Design review of the part built by this model. Coordinates are the model's own, in mm. Face numbers are marked on the shaded views. A direction names the side the tool comes from. Round coordinates to 2 decimals unless told otherwise and drop trailing zeros. Loops run counter-clockwise (first coordinate to the right, second up) from the corner with the lowest first, then second, coordinate; pieces in that order, holes last. Notation, with made-up numbers: (79, -8) - (136, -8) arc R12 cw to (136, 3) - close; hole circle Ø5 at (22, 81). An arc over 180 degrees is marked (long way). Use one line per item in the form item = value. Start each with the question number.
(1) We need section D-D, the plane z = -0.75. Write out the cut boundary in (x, y) (3 decimals).
(2) The part is to be moulded in two halves that separate along X. For the marked faces 3, 4, 5 and 6, say which applies: released by +X, released by -X, zero draft, split by the parting line, or undercut.
(3) We need section C-C, the plane z = 1. Write out the cut boundary in (x, y).
(4) We need section B-B, the plane x = 0. Write out the cut boundary in (y, z) (3 decimals).
(5) We need section A-A, the plane y = 0. Write out the cut boundary in (x, z) (3 decimals).
(6) For pin 1 (1.5 mm diameter, centred on x = -4.5, y = 2, fed in from +Z), flat-tipped, find the tip position at first contact; note if it passes through.
(7) Machinability: for the marked faces 1 and 2, which of the approach directions +Z, -Z, +X, -X, +Y, -Y give a long, thin tool a straight path to every point of the face, cutting with its end or side? Answer none if there is none.
(8) Wall thickness on probe 1 along Y at (x, z) = (0, -1.05) (3 decimals); probe 2 along Z at (x, y) = (-0.5, -2.75); probe 3 along X at (y, z) = (4.25, 1.75): over which ranges is each line inside the solid? List them lowest first. Write a range as [from, to].
Autodesk Inventor part; units mm, degrees
ref_plane "YZ Plane" through (0, 0, 0) normal (1, 0, 0) x (0, 1, 0)
ref_plane "XZ Plane" through (0, 0, 0) normal (0, 1, 0) x (-1, 0, 0)
ref_plane "XY Plane" through (0, 0, 0) normal (0, 0, 1) x (1, 0, 0)
sketch "Sketch1" plane through (0, 0, 0) normal (0, 0, 1) x (1, 0, 0)
  circle A0 centre (0, 0) radius 2.075
  line L0 (-12.5, 5) -> (12.5, 5)
  line L1 (12.5, 5) -> (12.5, -5)
  line L2 (12.5, -5) -> (-12.5, -5)
  line L3 (-12.5, -5) -> (-12.5, 5)
  line L4 (-12.5, 5) -> (12.5, -5) construction
  line L5 (12.5, 5) -> (-12.5, -5) construction
  dimension "d0" = 4.15
  dimension "d1" = 25
  dimension "d2" = 10
extrude "Extrusion1" add sketch "Sketch1" against normal blind 3.5
sketch "Sketch3" plane through (0, 0, 0) normal (0, 0, 1) x (1, 0, 0)
  line L0 (-22.7487, 17.0919) -> (-7.9081, 2.2513)
  arc A0 (-7.3223, 0.837) -> (-7.9081, 2.2513) centre (-9.3223, 0.837) ccw
  line L1 (-7.3223, 0.837) -> (-7.3223, -0.837)
  arc A1 (-7.9081, -2.2513) -> (-7.3223, -0.837) centre (-9.3223, -0.837) ccw
  line L2 (-7.9081, -2.2513) -> (-22.7487, -17.0919)
  line L3 (22.7487, -17.0919) -> (7.9081, -2.2513)
  arc A2 (7.3223, -0.837) -> (7.9081, -2.2513) centre (9.3223, -0.837) ccw
  line L4 (7.3223, -0.837) -> (7.3223, 0.837)
  arc A3 (7.9081, 2.2513) -> (7.3223, 0.837) centre (9.3223, 0.837) ccw
  line L5 (7.9081, 2.2513) -> (22.7487, 17.0919)
  circle A4 centre (0, 0) radius 1.65
  line L6 (-22.7487, 17.0919) -> (-22.7487, -17.0919)
  line L7 (22.7487, 17.0919) -> (22.7487, -17.0919)
  line L8 (-8.0495, 2.1098) -> (-22.5487, 16.609)
  line L9 (-22.5487, 16.609) -> (-22.5487, -16.609)
  line L10 (-22.5487, -16.609) -> (-8.0495, -2.1098)
  arc A5 (-7.5223, 0.837) -> (-8.0495, 2.1098) centre (-9.3223, 0.837) ccw
  line L11 (-7.5223, 0.837) -> (-7.5223, -0.837)
  arc A6 (-8.0495, -2.1098) -> (-7.5223, -0.837) centre (-9.3223, -0.837) ccw
  line L12 (7.5223, -0.837) -> (7.5223, 0.837)
  arc A7 (8.0495, 2.1098) -> (7.5223, 0.837) centre (9.3223, 0.837) ccw
  line L13 (8.0495, 2.1098) -> (22.8902, 16.9505)
  line L14 (22.5487, 17.0919) -> (22.5487, -16.609)
  line L15 (22.5487, -16.609) -> (8.0495, -2.1098)
  arc A8 (7.5223, -0.837) -> (8.0495, -2.1098) centre (9.3223, -0.837) ccw
  line L16 (-12.5, -5) -> (12.5, -5)
  line L17 (12.5, -5) -> (12.5, 5)
  line L18 (12.5, 5) -> (-12.5, 5)
  line L19 (-12.5, 5) -> (-12.5, -5)
  circle A9 centre (0, 0) radius 2.075
  point P0 (8.0495, -2.1098)
  point P1 (10.9397, -5)
  point P2 (10.9397, 5)
  point P3 (-10.9397, 5)
  point P4 (-10.9397, -5)
  point P5 (-8.0495, -2.1098)
  dimension "d1" = 25
  dimension "d5" = 0.2
  dimension "d6" = 0.2
  dimension "d7" = 0.2
  dimension "d8" = 0.2
  dimension "d9" = 0.2
  dimension "d10" = 0.2
  dimension "d11" = 0.2
  dimension "d12" = 0.2
  dimension "d13" = 0.2
extrude "Extrusion2" add sketch "Sketch3" along normal blind 3 contours L8 A5 L11 A6 L10 L16 L19 L18 | L18 L17 L16 L15 A8 L12 A7 L13
equation "\"d6\" = d5"
equation "\"d7\" = d5"
equation "\"d8\" = d5"
equation "\"d9\" = d5"
equation "\"d10\" = d5"
equation "\"d11\" = d5"
equation "\"d12\" = d5"
equation "\"d13\" = d5"
properties part number "backing_nut"
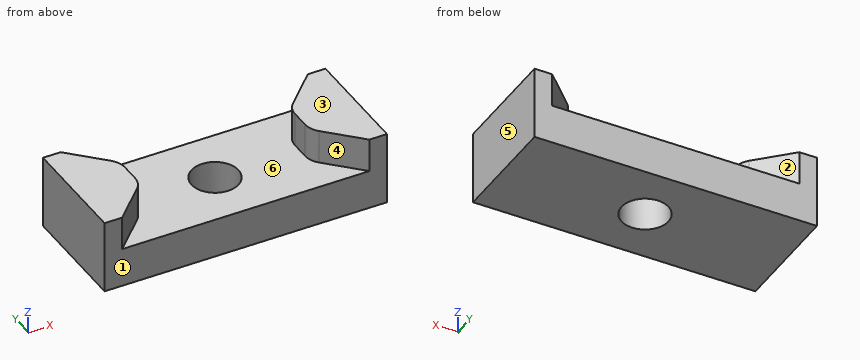
Data:
q1.outline = (-12.5, -5) - (12.5, -5) - (12.5, 5) - (-12.5, 5) - close; hole circle Ø4.15 at (0, 0)
q2.face_3 = zero draft
q2.face_4 = undercut
q2.face_5 = released by +X
q2.face_6 = undercut
q3.outline = (-12.5, -5) - (-10.94, -5) - (-8.05, -2.11) arc R1.8 ccw to (-7.52, -0.84) - (-7.52, 0.84) arc R1.8 ccw to (-8.05, 2.11) - (-10.94, 5) - (-12.5, 5) - close; (7.52, -0.84) arc R1.8 ccw to (8.05, -2.11) - (10.94, -5) - (12.5, -5) - (12.5, 5) - (10.94, 5) - (8.05, 2.11) arc R1.8 ccw to (7.52, 0.84) - close
q4.outline = (-5, -3.5) - (-2.075, -3.5) - (-2.075, 0) - (-5, 0) - close; (2.075, -3.5) - (5, -3.5) - (5, 0) - (2.075, 0) - close
q5.outline = (-12.5, -3.5) - (-2.075, -3.5) - (-2.075, 0) - (-7.522, 0) - (-7.522, 3) - (-12.5, 3) - close; (2.075, -3.5) - (12.5, -3.5) - (12.5, 3) - (7.522, 3) - (7.522, 0) - (2.075, 0) - close
q6.pin_1 = 0
q7.face_1 = +Z, -Z, +X, -X, -Y
q7.face_2 = +Z, +Y
q8.probe_1 = [-5, -2.075], [2.075, 5]
q8.probe_2 = [-3.5, 0]
q8.probe_3 = [-12.5, -10.19], [10.19, 12.5]
